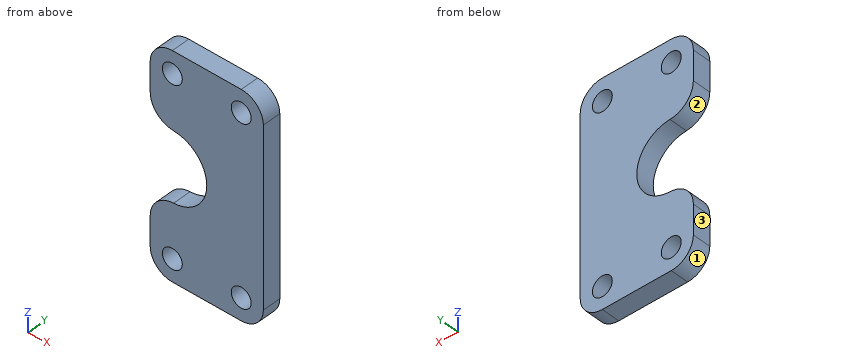
Autodesk Inventor part; units mm, degrees
ref_plane "YZ Plane" through (0, 0, 0) normal (1, 0, 0) x (0, 1, 0)
ref_plane "XZ Plane" through (0, 0, 0) normal (0, 1, 0) x (-1, 0, 0)
ref_plane "XY Plane" through (0, 0, 0) normal (0, 0, 1) x (1, 0, 0)
sketch "Sketch1" plane through (0, 0, 0) normal (0, 1, 0) x (-1, 0, 0)
  circle A0 centre (0, 0) radius 2.6
  circle A1 centre (-18, 0) radius 2.6
  circle A2 centre (0, -46) radius 2.6
  circle A3 centre (-18, -46) radius 2.6
  circle A4 centre (0, -23) radius 9 construction
  circle A5 centre (0, 0) radius 5.775 construction
  circle A6 centre (0, -46) radius 5.775 construction
  circle A7 centre (-18, -46) radius 5.775 construction
  circle A8 centre (-18, 0) radius 5.775 construction
  line L0 (5.775, 0) -> (5.775, -7.6608)
  line L1 (5.775, -46) -> (5.775, -38.3392)
  arc A9 (5.775, -38.3392) -> (-0.3371, -31.9937) centre (-0.575, -38.3392) ccw
  arc A10 (-0.3371, -14.0063) -> (5.775, -7.6608) centre (-0.575, -7.6608) ccw
  arc A11 (-0.3371, -14.0063) -> (-0.3371, -31.9937) centre (0, -23) ccw
  line L2 (-23.775, 0) -> (-23.775, -46)
  line L3 (0, -51.775) -> (-18, -51.775)
  line L4 (0, 5.775) -> (-18, 5.775)
  arc A12 (5.775, 0) -> (0, 5.775) centre (0, 0) ccw
  arc A13 (-18, 5.775) -> (-23.775, 0) centre (-18, 0) ccw
  arc A14 (0, -51.775) -> (5.775, -46) centre (0, -46) ccw
  arc A15 (-23.775, -46) -> (-18, -51.775) centre (-18, -46) ccw
  dimension "d0" = 5.2
  dimension "d1" = 18
  dimension "d2" = 46
  dimension "d3" = 18
  dimension "d4" = 23
  dimension "d5" = 3.175
  dimension "d6" = 6.35
extrude "Extrusion1" add sketch "Sketch1" along normal blind 4.7625
properties part number "CNC-002-ShimStructureGusset2" material "ABS Plastic"
The model under review builds one solid part; all positions refer to its coordinate system, in mm. Face numbers are marked on the shaded views. Coordinates: 2 decimals unless noted, no trailing zeros. Write each loop counter-clockwise with the first axis right and the second up, starting at its lowest first coordinate (ties: lowest second). Pieces come first, ordered by that corner, then holes.
1) To check wall thickness, follow probe 1 along Z at (x, y) = (18, 3.85) (3 decimals); probe 2 along Z at (x, y) = (0.5, 3.7) (3 decimals); probe 3 along X at (y, z) = (1.65, -48). State the ranges of each line that lie inside material, in increasing order.
2) The part is to be moulded in two halves that separate along Z. For the marked faces 1, 2 and 3, say which applies: pulls with the +Z half, pulls with the -Z half, needs draft (parallel to the pull), parting line crosses it, or undercut.
3) We need section D-D on z = -23. State the section outline as (x, y) points (1 decimal), then the cut area to 3 significant figures.
4) We need section C-C on z = -47. State the section outline as (x, y) points.
5) We need section B-B on x = 4.25. State the section outline as (y, z) points (1 decimal), then the cut area to 3 significant figures.
6) We need section A-A on y = 3.3. State the section outline as (x, z) points (3 decimals).
Answer list:
1. probe 1: z = -51.775 to -48.6, -43.4 to -2.6, 2.6 to 5.775
1. probe 2: z = -51.775 to -48.551, -43.449 to -31.986, -14.014 to -2.551, 2.551 to 5.775
1. probe 3: x = -5.42 to -1.66, 1.66 to 16.34, 19.66 to 23.42
2. face 1: pulls with the -Z half
2. face 2: undercut
2. face 3: needs draft
3. outline: (9, 0) - (23.8, 0) - (23.8, 4.8) - (9, 4.8) - close
3. area: 70.4 mm2
4. outline: (-5.69, 0) - (-2.4, 0) - (-2.4, 4.76) - (-5.69, 4.76) - close; (2.4, 0) - (15.6, 0) - (15.6, 4.76) - (2.4, 4.76) - close; (20.4, 0) - (23.69, 0) - (23.69, 4.76) - (20.4, 4.76) - close
5. outline: (0, -51.8) - (4.8, -51.8) - (4.8, -30.9) - (0, -30.9) - close; (0, -15.1) - (4.8, -15.1) - (4.8, 5.8) - (0, 5.8) - close
5. area: 199 mm2
6. outline: (-5.775, -46) arc R5.775 ccw to (0, -51.775) - (18, -51.775) arc R5.775 ccw to (23.775, -46) - (23.775, 0) arc R5.775 ccw to (18, 5.775) - (0, 5.775) arc R5.775 ccw to (-5.775, 0) - (-5.775, -7.661) arc R6.35 ccw to (0.337, -14.006) arc R9 cw to (0.337, -31.994) arc R6.35 ccw to (-5.775, -38.339) - close; hole circle Ø5.2 at (0, -46); hole circle Ø5.2 at (0, 0); hole circle Ø5.2 at (18, -46); hole circle Ø5.2 at (18, 0)
